Geometry check sheet. Reference: the model listing, model coordinates, mm. A direction names the side the tool comes from. Coordinates: 2 decimals unless noted, no trailing zeros. Order: outer loops, then holes, each group sorted by start corner. A loop starts at its lowest first (then second) coordinate and runs counter-clockwise, first axis right, second up. Notation, with made-up numbers: (48.5, -21.75) - (104.5, -21.75) arc R33 cw to (104.5, 14.25) - close; hole circle Ø6 at (51, 48). An arc over 180 degrees is marked (long way). One line per item, written item: value. Start each with the question number.
```python
from build123d import *

# Parameters (mm, degrees)
BOSS_EXTRUDE1_DEPTH = 8.0518
SKETCH2_R           = 13.39215
BOSS_EXTRUDE2_DEPTH = 20.2438
SKETCH3_R           = 5.8039
CUT_EXTRUDE1_DEPTH  = 10.3886
SKETCH4_R           = 8.0137
CUT_EXTRUDE2_DEPTH  = 16.1925


with BuildPart() as part:
    # Sketch1 → Boss-Extrude1 (new body)
    with BuildSketch(Plane(origin=(0, 0, 0), x_dir=(1, 0, 0), z_dir=(0, 1, 0))):
        Polygon((18.22088582, 0), (9.11044291, 15.77975), (-9.11044291, 15.77975), (-18.22088582, 0), (-9.11044291, -15.77975), (9.11044291, -15.77975), align=None)
    extrude(amount=BOSS_EXTRUDE1_DEPTH)

    # Sketch2 → Boss-Extrude2 (add)
    with BuildSketch(Plane(origin=(0, 0, 0), x_dir=(-1, 0, 0), z_dir=(0, -1, 0))):
        with Locations(Location((0, 0, 0), (0, 0, 90))):
            Circle(SKETCH2_R)
    extrude(amount=BOSS_EXTRUDE2_DEPTH)

    # Sketch3 → Cut-Extrude1 (cut)
    with BuildSketch(Plane(origin=(0, 8.0518, 0), x_dir=(1, 0, 0), z_dir=(0, 1, 0))):
        with Locations(Location((0, 0, 0), (0, 0, 270))):
            Circle(SKETCH3_R)
    extrude(amount=-CUT_EXTRUDE1_DEPTH, mode=Mode.SUBTRACT)

    # Sketch4 → Cut-Extrude2 (cut)
    with BuildSketch(Plane.XZ.offset(20.2438)):
        with Locations(Location((0, 0, 0), (0, 0, 270))):
            Circle(SKETCH4_R)
    extrude(amount=-CUT_EXTRUDE2_DEPTH, mode=Mode.SUBTRACT)

    # Sketch5 → Cut-Revolve4 (revolve, cut)
    with BuildSketch(Plane.XY, mode=Mode.PRIVATE) as cut_revolve4_sk:
        Polygon((0, -2.3368), (0, -4.0513), (-8.0137, -4.0513), (-5.8039, -2.3368), align=None)
    revolve(cut_revolve4_sk.sketch.rotate(Axis((0, -2.3368, 0), (0, -1, 0)), 270), axis=Axis((0, -2.3368, 0), (0, -1, 0)), mode=Mode.SUBTRACT)


solid = part.part
```
Q1. Cross-section at D-D, the plane x = -10. Enter the section's corners in (y, z).
Q2. Material ranges on probe 1 along X at (y, z) = (-9, 0); probe 2 along X at (y, z) = (1.5, 0); probe 3 along Z at (x, y) = (-5.5, -4.5), recorded low to high.
Q3. Cross-section at C-C, the plane z = 9. Enter the section's corners in (x, y), and give its area (3 significant figures).
Q4. Cross-section at A-A, the plane x = 0. Enter the section's corners in (y, z).
Q5. Cross-section at B-B, the plane y = 2. Enter the section's corners in (x, z).
Q6. Set-up check for faces 5 (the flat face through (13.73, 3.97, -7.78)), 6 (the cylindrical face through (-13.074, -9.98, 2.903)): record each of +Z, -Z, +X, -X, +Y, -Y from which the full face is reachable in a straight line by a thin tool's end or side.
Q7. Release check for a two-part mould opening along X. For faces 1 (the flat face through (-13.6, 4, -8)), 2 (the cylindrical face through (1.743, 2.93, 5.536)), 3 (the cylindrical face through (-4.876, -12.261, 6.359)), 4 (the flat face through (8, 8.052, 0)) record: released by +X, released by -X, zero draft, split by the parting line, or undercut.
Q8. Gauge pin test, flat ends, axial feed: P1, Ø3, axis at x = 11.5, y = -14.5, coming from the +Z side; P2, Ø10, axis at y = -9.5, z = 0.5, coming from the +X side; P3, Ø2, axis at x = 11.5, z = 9.5, coming from the -Y side. Record the tip position at first contact, or that the pin passes through.
Check result:
1. outline: (-20.24, -8.91) - (0, -8.91) - (0, -14.24) - (8.05, -14.24) - (8.05, 14.24) - (0, 14.24) - (0, 8.91) - (-20.24, 8.91) - close
2. probe 1: x = -13.39 to -8.01, 8.01 to 13.39
2. probe 2: x = -18.22 to -5.8, 5.8 to 18.22
2. probe 3: z = -12.21 to -5.83, 5.83 to 12.21
3. outline: (-13.02, 0) - (-9.92, 0) - (-9.92, -20.24) - (9.92, -20.24) - (9.92, 0) - (13.02, 0) - (13.02, 8.05) - (-13.02, 8.05) - close
3. area: 611 mm2
4. outline: (-20.24, -13.39) - (0, -13.39) - (0, -15.78) - (8.05, -15.78) - (8.05, -5.8) - (-2.34, -5.8) - (-4.05, -8.01) - (-20.24, -8.01) - close; (-20.24, 8.01) - (-4.05, 8.01) - (-2.34, 5.8) - (8.05, 5.8) - (8.05, 15.78) - (0, 15.78) - (0, 13.39) - (-20.24, 13.39) - close
5. outline: (-18.22, 0) - (-9.11, -15.78) - (9.11, -15.78) - (18.22, 0) - (9.11, 15.78) - (-9.11, 15.78) - close; hole circle Ø11.61 at (0, 0)
6. face 5: -Z, +X, +Y, -Y
6. face 6: -Y
7. face 1: released by -X
7. face 2: undercut
7. face 3: undercut
7. face 4: zero draft
8. P1: stops at z = 8.91
8. P2: stops at x = 13.39
8. P3: stops at y = 0
